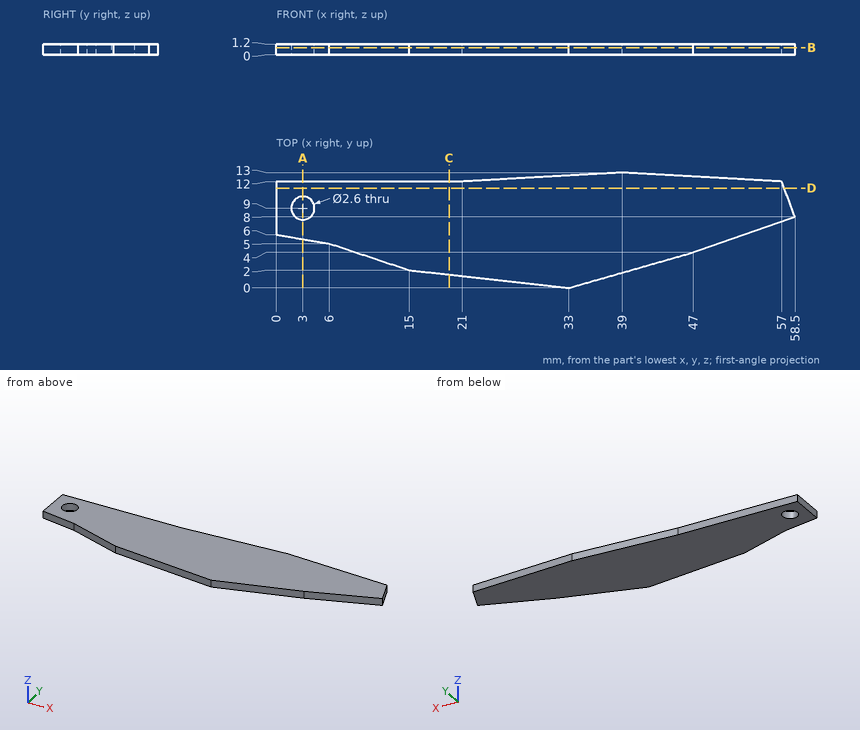
Source: three-view drawing plus pictorial views. Frame: mm from the lowest corner of the part. Round coordinates to 2 decimals unless told otherwise and drop trailing zeros. Write each loop counter-clockwise with the first axis right and the second up, starting at its lowest first coordinate (ties: lowest second). Pieces come first, ordered by that corner, then holes. Notation, with made-up numbers: M 32.25,6.5 L 40.25,6.5 A7 cw 40.25,10.5 Z; hole C 44,-8.5 d1. An arc over 180 degrees is marked long. Write item = value, one per line.
Item 1: Pin query (flat end, axial travel): P1, Ø0.6, axis at x = 6.5, z = 0.5, coming from the +Y side. Return the tip coordinate at first contact, or that it passes through.
Findings:
P1 = 12
Item 2: Material intervals for line 1 along Y through (x, z) = (3, 0.65); line 2 along Y through (x, z) = (27, 0.95); line 3 along Y through (x, z) = (28, 0.25), sorted ascending. Write a range as [from, to].
Findings:
line_1 = [5.5, 7.7], [10.3, 12]
line_2 = [0.67, 12.33]
line_3 = [0.56, 12.39]
Item 3: Section query B-B on z = 0.8. Return loops of the section in (x, y).
Findings:
outline = M 0,6 L 6,5 L 15,2 L 33,0 L 47,4 L 58.5,8 L 57,12 L 39,13 L 21,12 L 0,12 Z; hole C 3,9 d2.6
Item 4: Section query A-A on x = 3. Return loops of the section in (y, z).
Findings:
outline = M 5.5,0 L 7.7,0 L 7.7,1.2 L 5.5,1.2 Z; M 10.3,0 L 12,0 L 12,1.2 L 10.3,1.2 Z
Item 5: Section query D-D on y = 11.25. Return loops of the section in (x, z), then the cut area to 3 significant figures.
Findings:
outline = M 0,0 L 57.28,0 L 57.28,1.2 L 0,1.2 Z
area = 68.7 mm^2
Item 6: Section query C-C on x = 19.5. Return loops of the section in (y, z), then the cut area to 3 significant figures.
Findings:
outline = M 1.5,0 L 12,0 L 12,1.2 L 1.5,1.2 Z
area = 12.6 mm^2
